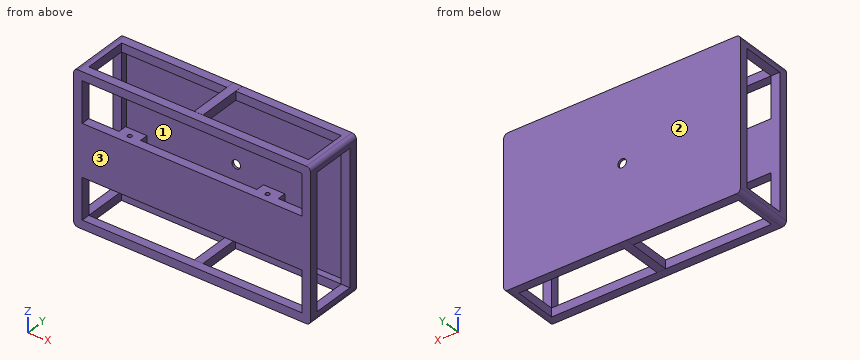
from build123d import *

# Parameters (mm, degrees)
SKETCH1_W           = 550
SKETCH1_H           = 350
SKETCH1_W_2         = 510
SKETCH1_H_2         = 310
BOSS_EXTRUDE1_DEPTH = 20
SKETCH3_W           = 20
SKETCH3_H           = 20
SKETCH3_W_2         = 20.022451752
SKETCH3_H_2         = 20.022451752
SKETCH3_W_3         = 20.433308148
SKETCH3_H_3         = 20.433308148
BOSS_EXTRUDE2_DEPTH = 120
SKETCH4_W           = 550
SKETCH4_H           = 350
SKETCH4_W_2         = 510
SKETCH4_H_2         = 310
BOSS_EXTRUDE3_DEPTH = 20
SKETCH5_W           = 550
SKETCH5_H           = 350
BOSS_EXTRUDE4_DEPTH = 5
SKETCH6_W           = 550
SKETCH6_H           = 120
BOSS_EXTRUDE5_DEPTH = 20
SKETCH7_W           = 49.868309686
SKETCH7_H           = 40
SKETCH7_W_2         = 49.961884124
BOSS_EXTRUDE6_DEPTH = 120
SKETCH8_R           = 5
CUT_EXTRUDE1_DEPTH  = 181
FILLET1_R           = 10
SKETCH9_R           = 10
CUT_EXTRUDE2_DEPTH  = 43


with BuildPart() as part:
    # Sketch1 → Boss-Extrude1 (new body)
    with BuildSketch(Plane(origin=(0, 0, 0), x_dir=(1, 0, 0), z_dir=(0, 1, 0))):
        Rectangle(SKETCH1_W, SKETCH1_H)
        Rectangle(SKETCH1_W_2, SKETCH1_H_2, mode=Mode.SUBTRACT)
    extrude(amount=BOSS_EXTRUDE1_DEPTH)

    # Sketch3 → Boss-Extrude2 (add)
    with BuildSketch(Plane(origin=(0, 20, 0), x_dir=(1, 0, 0), z_dir=(0, 1, 0))):
        with Locations((-265, 165)):
            Rectangle(SKETCH3_W, SKETCH3_H)
        with Locations((-265, -165)):
            Rectangle(SKETCH3_W, SKETCH3_H)
        with Locations((265, -165)):
            Rectangle(SKETCH3_W, SKETCH3_H)
        with Locations((265, 165)):
            Rectangle(SKETCH3_W, SKETCH3_H)
        with Locations((0, 165)):
            Rectangle(SKETCH3_W_2, SKETCH3_H_2)
        with Locations((0, -165)):
            Rectangle(SKETCH3_W_3, SKETCH3_H_3)
    extrude(amount=BOSS_EXTRUDE2_DEPTH)

    # Sketch4 → Boss-Extrude3 (add)
    with BuildSketch(Plane(origin=(0, 140, 0), x_dir=(1, 0, 0), z_dir=(0, 1, 0))):
        Rectangle(SKETCH4_W, SKETCH4_H)
        Rectangle(SKETCH4_W_2, SKETCH4_H_2, mode=Mode.SUBTRACT)
    extrude(amount=-BOSS_EXTRUDE3_DEPTH)

    # Sketch5 → Boss-Extrude4 (add)
    with BuildSketch(Plane(origin=(0, 140, 0), x_dir=(1, 0, 0), z_dir=(0, 1, 0))):
        Rectangle(SKETCH5_W, SKETCH5_H)
    extrude(amount=-BOSS_EXTRUDE4_DEPTH)

    # Sketch6 → Boss-Extrude5 (add)
    with BuildSketch(Plane.XZ):
        Rectangle(SKETCH6_W, SKETCH6_H)
    extrude(amount=-BOSS_EXTRUDE5_DEPTH)

    # Sketch7 → Boss-Extrude6 (add)
    with BuildSketch(Plane.XY.offset(60)):
        with Locations((-159.939483021, 20)):
            Rectangle(SKETCH7_W, SKETCH7_H)
        with Locations((160.017500796, 20)):
            Rectangle(SKETCH7_W_2, SKETCH7_H)
    extrude(amount=-BOSS_EXTRUDE6_DEPTH)

    # Sketch8 → Cut-Extrude1 (cut)
    with BuildSketch(Plane.XY.offset(60)):
        with Locations((160.017500796, 20)):
            Circle(SKETCH8_R)
        with Locations((-159.939483021, 20)):
            Circle(SKETCH8_R)
    extrude(amount=-CUT_EXTRUDE1_DEPTH, mode=Mode.SUBTRACT)

    # Fillet1
    fillet1_edges = [part.edges().sort_by_distance(p)[0] for p in [
        (275, 70, 175),
        (-275, 70, 175),
        (-275, 70, -175),
        (275, 70, -175),
    ]]
    fillet(fillet1_edges, radius=FILLET1_R)

    # Sketch9 → Cut-Extrude2 (cut)
    with BuildSketch(Plane(origin=(0, 140, 0), x_dir=(1, 0, 0), z_dir=(0, 1, 0))):
        with Locations(Location((0, 0, 0), (0, 0, 270))):
            Circle(SKETCH9_R)
    extrude(amount=-CUT_EXTRUDE2_DEPTH, mode=Mode.SUBTRACT)


solid = part.part
Verification items for the finished model (mm, model axes). Face numbers are marked on the shaded views. Round coordinates to 2 decimals unless told otherwise and drop trailing zeros. Order: outer loops, then holes, each group sorted by start corner. A loop starts at its lowest first (then second) coordinate and runs counter-clockwise, first axis right, second up.
1. Go/stop test with flat-tipped pins: P1, Ø6, axis at x = -116, z = -72, coming from the -Y side; P2, Ø16, axis at y = 30.5, z = 26.5, coming from the +X side; P3, Ø8, axis at y = 44.5, z = 60, coming from the -X side; P4, Ø4.5, axis at x = -136.5, y = 130, coming from the +Z side. Record where each tip stops, or that it passes through.
Final values:
P1: stops at y = 135
P2: stops at x = 185
P3: passes through
P4: stops at z = 175
2. Thickness scan on L1, parallel to Z at x = -20.5, y = 6.5; L2, parallel to Y at x = 2.5, z = -19.5; L3, parallel to X at y = 132.5, z = 79. Record the ranges inside material, lowest first.
Final values:
L1: z = -175 to -155, -60 to 60, 155 to 175
L2: y = 0 to 20, 135 to 140
L3: x = -275 to -255, 255 to 275
3. Section check A-A on z = 33.5. Record the cut outline in (x, y), then the cut area to 3 significant figures.
Final values:
outline: (-275, 0) - (275, 0) - (275, 20) - (185, 20) - (185, 40) - (135.04, 40) - (135.04, 20) - (-135.01, 20) - (-135.01, 40) - (-184.87, 40) - (-184.87, 20) - (-275, 20) - close; (-275, 120) - (-255, 120) - (-255, 135) - (255, 135) - (255, 120) - (275, 120) - (275, 140) - (-275, 140) - close; hole circle Ø10 at (-159.94, 20); hole circle Ø10 at (160.02, 20)
area: 16,200 mm2
4. Release check for a two-part mould opening along Y. For the marked faces 1, 2 and 3 record: +Y half, -Y half, draft (parallel to the pull), parting line (faces both ways), or undercut.
Final values:
face 1: undercut
face 2: +Y half
face 3: -Y half
5. Section check C-C on x = 0. State how many separate pieces and enclosed holes the cut face has, then the cut area to 3 significant figures.
Final values:
separate pieces: 3
enclosed holes: 0
area: 9,500 mm2
6. Section check D-D on z = 142.5. Record the cut outline in (x, y).
Final values:
outline: (-275, 0) - (-255, 0) - (-255, 20) - (-275, 20) - close; (-275, 120) - (-255, 120) - (-255, 135) - (255, 135) - (255, 120) - (275, 120) - (275, 140) - (-275, 140) - close; (255, 0) - (275, 0) - (275, 20) - (255, 20) - close
7. Section check B-B on x = 236.5. Record the cut outline in (y, z).
Final values:
outline: (0, -175) - (20, -175) - (20, -155) - (0, -155) - close; (0, -60) - (20, -60) - (20, 60) - (0, 60) - close; (0, 155) - (20, 155) - (20, 175) - (0, 175) - close; (120, -175) - (140, -175) - (140, 175) - (120, 175) - (120, 155) - (135, 155) - (135, -155) - (120, -155) - close
